Job drawing, mm, ordinate dimensions from the low corner. One solid piece. A direction names the side the tool comes from. Give positions to 0.01 mm unless a question says otherwise; leave off trailing zeros. Order: outer loops, then holes, each group sorted by start corner. A loop starts at its lowest first (then second) coordinate and runs counter-clockwise, first axis right, second up.
1. Drop flat-ended pins along their axis: pin 1 Ø7.5 at (x, y) = (71, 60.5) entering from -Z; pin 2 Ø4 at (x, y) = (42.5, 30.5) entering from -Z; pin 3 Ø9 at (x, z) = (74.5, 7.5) entering from +Y. Give the stop position or say it passes through.
2. Slice it at B-B on y = 48.5. List the corners of the cut face in (x, z).
3. Slice it at C-C on x = 62. List the corners of the cut face in (y, z).
4. Slice it at A-A on x = 93. List the corners of the cut face in (y, z), and give its area (3 significant figures).
5. Slice it at D-D on z = 15. List the corners of the cut face in (x, y) (3 decimals).
6. Probe line 1 (X direction, y = 63, z = 25.5); line 2 (Z direction, x = 55.5, y = 16); line 3 (Y direction, x = 17.5, z = 24). List the from-to ranges inside material, lowest first.
7. Mould opens along X. For the marked faces 1, 2, 3 and 4 say: +X half, -X half, draft (parallel to the pull), parting line (faces both ways), or undercut.
8. Which spindle directions (+Z, -Z, +X, -X, +Y, -Y) get a long thin tool onto all of the face, cutting with end or side? Do the marked faces 5, 6, 7 and 8. Say none if no direction does.
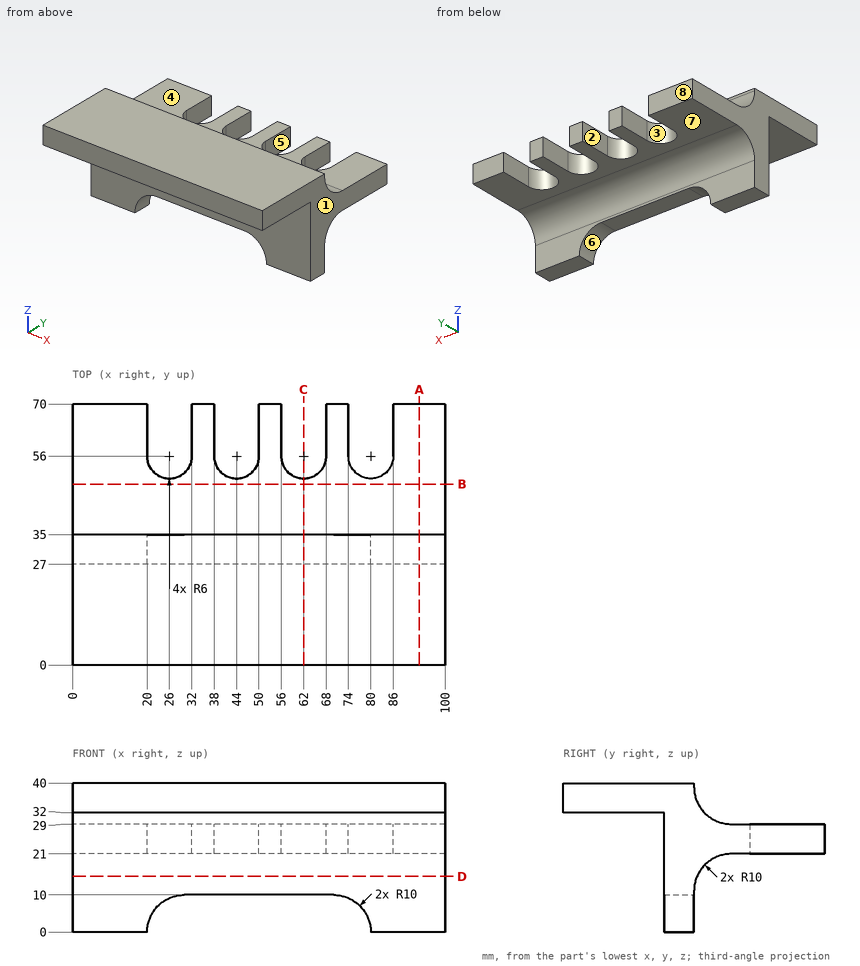
Data:
1. pin 1: stops at z = 21
1. pin 2: stops at z = 10
1. pin 3: stops at y = 35.05
2. outline: (0, 21) - (100, 21) - (100, 29) - (0, 29) - close
3. outline: (0, 32) - (27, 32) - (27, 10) - (35, 10) - (35, 11) arc R10 cw to (45, 21) - (50, 21) - (50, 29) - (45, 29) arc R10 cw to (35, 39) - (35, 40) - (0, 40) - close
4. outline: (0, 32) - (27, 32) - (27, 0) - (35, 0) - (35, 11) arc R10 cw to (45, 21) - (70, 21) - (70, 29) - (45, 29) arc R10 cw to (35, 39) - (35, 40) - (0, 40) - close
4. area: 859 mm2
5. outline: (0, 27) - (100, 27) - (100, 35.835) - (0, 35.835) - close
6. line 1: x = 0 to 20, 32 to 38, 50 to 56, 68 to 74, 86 to 100
6. line 2: z = 32 to 40
6. line 3: y = 27 to 70
7. face 1: +X half
7. face 2: undercut
7. face 3: undercut
7. face 4: draft
8. face 5: +Z, -Z, +Y
8. face 6: -Z, +Y, -Y
8. face 7: -Z, +X, -X, +Y
8. face 8: +Z, -Z, +X, -X, +Y
